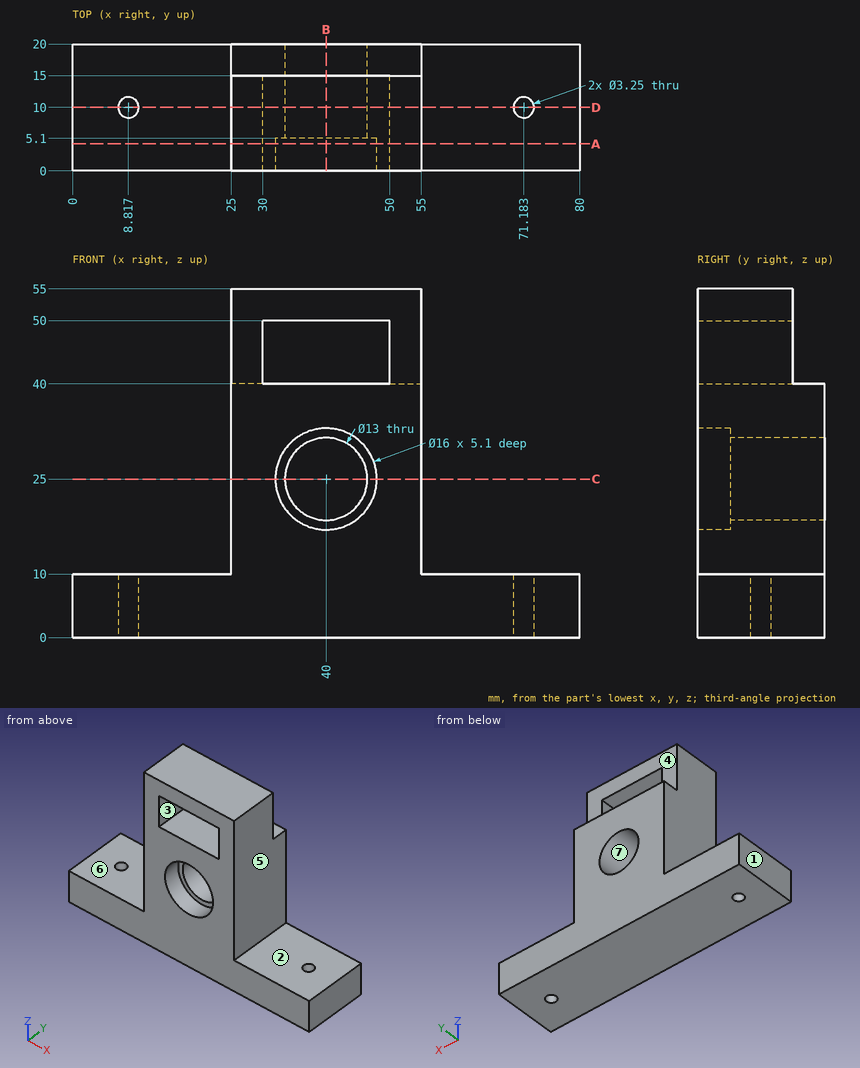
For this review, use the dimensioned drawing (mm, ordinates from the lowest corner) and the shaded views. A direction names the side the tool comes from. Coordinates: 2 decimals unless noted, no trailing zeros. Loops run counter-clockwise (first coordinate to the right, second up) from the corner with the lowest first, then second, coordinate; pieces in that order, holes last. Notation, with made-up numbers: (60, 83) -> (95, 83) arc R21 ccw to (95, 93) -> close; hole circle Ø6 at (85, -39.5). An arc over 180 degrees is marked (long way). Return JSON: item names as keys, results as strings. Group by question number.
(1) Consider section D-D, the plane y = 10. Give the boundary of the cut face in (x, z).
(2) Consider section B-B, the plane x = 40. Give the boundary of the cut face in (y, z).
(3) Consider section A-A, the plane y = 4.25. Give the boundary of the cut face in (x, z), plus the area to 3 significant figures.
(4) Consider section C-C, the plane z = 25. Give the boundary of the cut face in (x, y).
(5) To check wall thickness, follow L1, parallel to Z at x = 40, y = 2.15; L2, parallel to X at y = 10, z = 7; L3, parallel to X at y = 3.25, z = 42. State the ranges of each line that lie inside material, in increasing order.
(6) For pin 1 Ø11 at (y, z) = (6.5, 46.5) entering from -X; pin 2 Ø8 at (y, z) = (6, 46.5) entering from +X; pin 3 Ø10 at (x, y) = (62, 13) entering from +Z; pin 4 Ø2.5 at (x, y) = (71.183, 10) entering from +Z, all flat-tipped, find the tip position at first contact; note any pin that passes through.
(7) Tool access review of the marked faces 4, 5, 6 and 7: name each direction out of +Z, -Z, +X, -X, +Y, -Y from which nothing blocks a thin tool from reaching the whole face with its end or side.
(8) Mouldability with a two-part tool opening along Z and no side actions: class the marked faces 1, 2 and 3 as pulls with the +Z half, pulls with the -Z half, needs draft (parallel to the pull), parting line crosses it, or undercut.
Results below:
{
 "1": {"outline": "(0, 0) -> (7.19, 0) -> (7.19, 10) -> (0, 10) -> close; (10.44, 0) -> (69.56, 0) -> (69.56, 10) -> (55, 10) -> (55, 55) -> (25, 55) -> (25, 10) -> (10.44, 10) -> close; (72.81, 0) -> (80, 0) -> (80, 10) -> (72.81, 10) -> close; hole (30, 40) -> (50, 40) -> (50, 50) -> (30, 50) -> close; hole circle Ø13 at (40, 25)"},
 "2": {"outline": "(0, 0) -> (20, 0) -> (20, 18.5) -> (5.1, 18.5) -> (5.1, 17) -> (0, 17) -> close; (0, 33) -> (5.1, 33) -> (5.1, 31.5) -> (20, 31.5) -> (20, 40) -> (0, 40) -> close; (0, 50) -> (15, 50) -> (15, 55) -> (0, 55) -> close"},
 "3": {"outline": "(0, 0) -> (80, 0) -> (80, 10) -> (55, 10) -> (55, 55) -> (25, 55) -> (25, 10) -> (0, 10) -> close; hole (30, 40) -> (50, 40) -> (50, 50) -> (30, 50) -> close; hole circle Ø16 at (40, 25)", "area": "1,750 mm2"},
 "4": {"outline": "(25, 0) -> (32, 0) -> (32, 5.1) -> (33.5, 5.1) -> (33.5, 20) -> (25, 20) -> close; (46.5, 5.1) -> (48, 5.1) -> (48, 0) -> (55, 0) -> (55, 20) -> (46.5, 20) -> close"},
 "5": {"L1": "z = 0 to 17, 33 to 40, 50 to 55", "L2": "x = 0 to 7.19, 10.44 to 69.56, 72.81 to 80", "L3": "x = 25 to 30, 50 to 55"},
 "6": {"pin 1": "stops at x = 25", "pin 2": "stops at x = 55", "pin 3": "stops at z = 10", "pin 4": "passes through"},
 "7": {"face 4": "+Z, +X, -X, +Y", "face 5": "+Z, +X, +Y, -Y", "face 6": "+Z, -X, +Y, -Y", "face 7": "+Y, -Y"},
 "8": {"face 1": "needs draft", "face 2": "pulls with the +Z half", "face 3": "undercut"}
}
